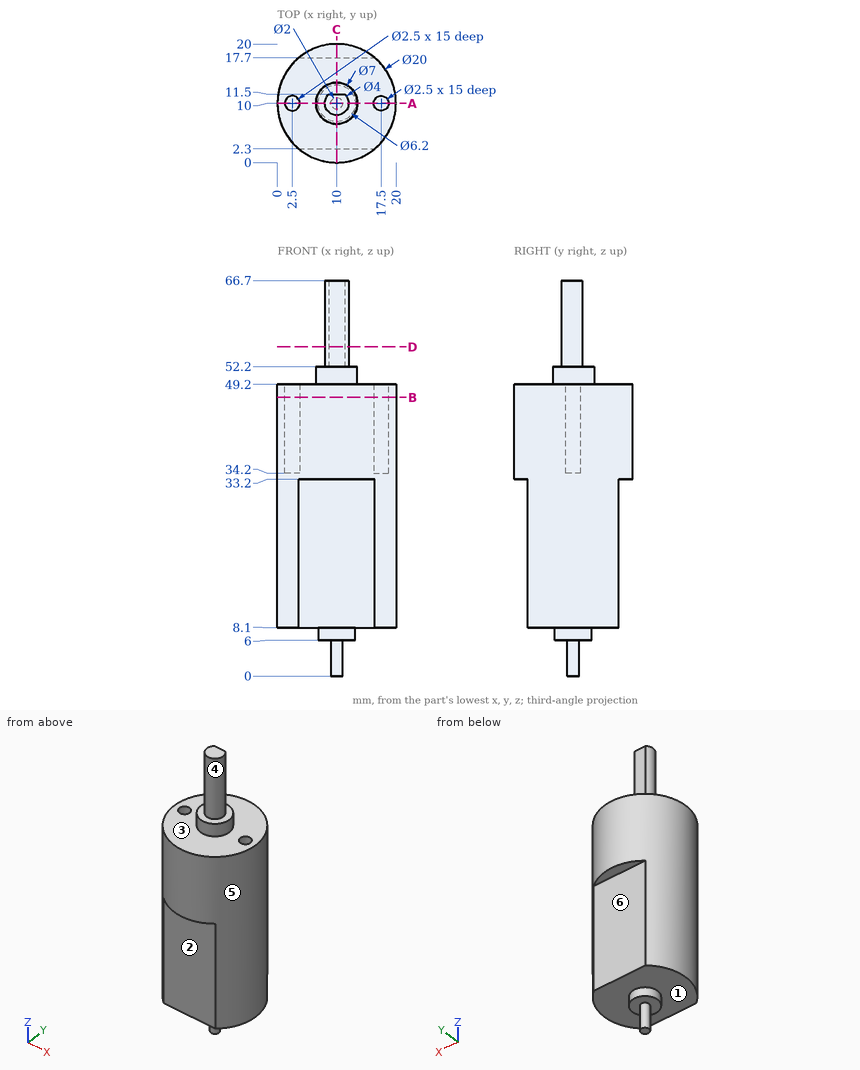
Answer from the drawing. Dimensions are ordinates in mm from the lowest x, y and z of the part. A direction names the side the tool comes from. Give positions to 0.01 mm unless a question says otherwise; leave off trailing zeros. Order: outer loops, then holes, each group sorted by start corner. A loop starts at its lowest first (then second) coordinate and runs counter-clockwise, first axis right, second up. Notation, with made-up numbers: (75.5, 38) -> (119.5, 38) arc R27 ccw to (119.5, 56) -> close; hole circle Ø10 at (6, -5.75). An arc over 180 degrees is marked (long way). One line per item, written item: value. Start each with the question number.
(1) The part is cut by section A-A (y = 10). Determine the outline of the cut face in (x, z), and give its area (3 significant figures).
(2) For a pull along Z with two mould halves and no side action, classify the marked faces 1, 2 and 3 as released by +Z, released by -Z, zero draft, split by the parting line, or undercut.
(3) The part is cut by section D-D (z = 55.5). Determine the outline of the cut face in (x, y), and give its area (3 significant figures).
(4) The part is cut by section C-C (x = 10). Determine the outline of the cut face in (y, z), and give its area (3 significant figures).
(5) A tool of negligible diameter and unlimited length cuts with its end or side. For the marked faces 4, 5 and 6, from which of +Z, -Z, +X, -X, +Y, -Y can it reach the whole face along a straight path? Write none if from no direction.
(6) The part is cut by section B-B (z = 47). Determine the outline of the cut face in (x, y).
(7) Flat-ended cylindrical pins translate along their axes: P1, Ø2, axis at x = 4, z = 46, coming from the -Y side; P2, Ø1.5, axis at y = 13, z = 27.5, coming from the +X side; P3, Ø8, axis at x = 6.5, z = 12, coming from the +Y side; P4, Ø5, axis at x = 10.5, y = 9.5, coming from the -Z side. Find the tip coordinate at first contact, or state that the pin passes through.
(8) Straight lines are drawn through the part: L1, parallel to Z at x = 12.5, y = 11.5; L2, parallel to Z at x = 7.25, y = 17.5; L3, parallel to Y at x = 17.5, z = 41. For each, find the intervals that lie inside material, in ascending order.
Taken from the geometry:
1. outline: (0, 8.1) -> (6.9, 8.1) -> (6.9, 6) -> (9, 6) -> (9, 0) -> (11, 0) -> (11, 6) -> (13.1, 6) -> (13.1, 8.1) -> (20, 8.1) -> (20, 49.2) -> (18.75, 49.2) -> (18.75, 34.2) -> (16.25, 34.2) -> (16.25, 49.2) -> (13.5, 49.2) -> (13.5, 52.2) -> (12, 52.2) -> (12, 66.7) -> (8, 66.7) -> (8, 52.2) -> (6.5, 52.2) -> (6.5, 49.2) -> (3.75, 49.2) -> (3.75, 34.2) -> (1.25, 34.2) -> (1.25, 49.2) -> (0, 49.2) -> close
1. area: 851 mm^2
2. face 1: released by -Z
2. face 2: zero draft
2. face 3: released by +Z
3. outline: (8.68, 11.5) arc R2 ccw (long way) to (11.32, 11.5) -> close
3. area: 11.7 mm^2
4. outline: (0, 33.2) -> (2.3, 33.2) -> (2.3, 8.1) -> (6.9, 8.1) -> (6.9, 6) -> (9, 6) -> (9, 0) -> (11, 0) -> (11, 6) -> (13.1, 6) -> (13.1, 8.1) -> (17.7, 8.1) -> (17.7, 33.2) -> (20, 33.2) -> (20, 49.2) -> (13.5, 49.2) -> (13.5, 52.2) -> (11.5, 52.2) -> (11.5, 66.7) -> (8, 66.7) -> (8, 52.2) -> (6.5, 52.2) -> (6.5, 49.2) -> (0, 49.2) -> close
4. area: 803 mm^2
5. face 4: +Z
5. face 5: +Z, -Z
5. face 6: -Z, +X, -X, +Y
6. outline: circle Ø20 at (10, 10); hole circle Ø2.5 at (2.5, 10); hole circle Ø2.5 at (17.5, 10)
7. P1: y = 1.34
7. P2: x = 19.74
7. P3: y = 17.7
7. P4: z = 0
8. L1: 6 to 52.2
8. L2: 8.1 to 49.2
8. L3: 3.39 to 8.75, 11.25 to 16.61
